Geometry: final body of the model. Coordinates: model frame, mm. Face numbers are marked on the shaded views. A direction names the side the tool comes from. Give positions to 0.01 mm unless a question says otherwise; leave off trailing zeros. Order: outer loops, then holes, each group sorted by start corner. A loop starts at its lowest first (then second) coordinate and runs counter-clockwise, first axis right, second up. Notation, with made-up numbers: (74.25, 76) - (111.25, 76) arc R27 cw to (111.25, 101) - close; hole circle Ø5 at (12.25, 17). An arc over 180 degrees is marked (long way). Use one line per item in the form item = value.
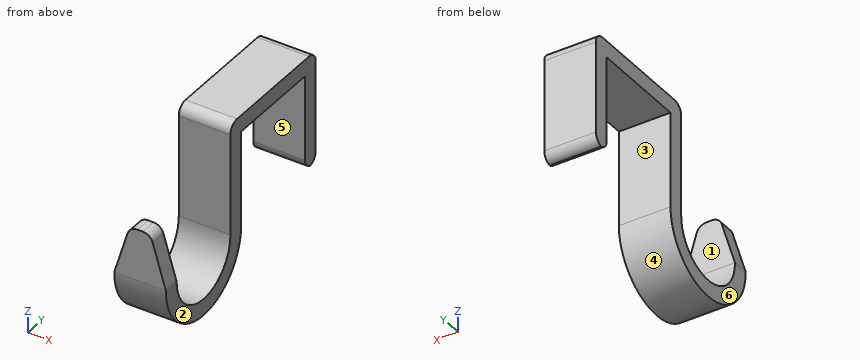
from build123d import *

# Parameters (mm, degrees)
F0_W        = 3.2
F0_H        = 10
F1_DEPTH    = 10
F2_SIZE2    = 10
F2_SIZE     = 3
F3_T1_DEPTH = 10.6403065089
F3_T3_DEPTH = 4.667688363
F3_T5_DEPTH = 20


# Not quite as in the source:
# - a fillet or chamfer that OpenCascade refuses, or shapes differently, is made with other operations: its cross-section is extruded or revolved along the edge and cut away or added


with BuildPart() as f1:
    # F0 (on Right) → F1 (new body)
    with BuildSketch(Plane.YZ):
        with Locations((-30.3, 5)):
            Rectangle(F0_W, F0_H)
        with BuildLine():
            Line((-9.5, 0), (-12.7, 0))
            ThreePointArc((-12.7, 0), (-20.7, -8), (-28.7, 0))
            Line((-28.7, 0), (-31.9, 0))
            ThreePointArc((-31.9, 0), (-20.7, -11.2), (-9.5, 0))
        make_face()
        Polygon((-12.7, 21.7), (-12.7, 0), (-9.5, 0), (-9.5, 18.5), (9.5, 18.5), (9.5, 0), (12.7, 0), (12.7, 21.7), align=None)
    extrude(amount=F1_DEPTH)

    # F2
    f2_edges = [f1.edges().sort_by_distance(p)[0] for p in [
        (10, -30.3, 10),
        (0, -30.3, 10),
    ]]
    f2_side = f1.faces().sort_by_distance((5, -30.3, 10))[0]
    chamfer(f2_edges, length=F2_SIZE, length2=F2_SIZE2, reference=f2_side)

    # F3: fillet of radius 2 on 8 edges, made by hand

    # F3_s2 → F3_t1 (cut)
    with BuildSketch(Plane.XZ.offset(24.9798467455)):
        with BuildLine():
            ThreePointArc((5.5119386982, 10), (6.7057997575, 9.6045858566), (7.4275912687, 8.5746957711))
            Line((7.4275912687, 8.5746957711), (7, 10))
            Line((7, 10), (5.5119386982, 10))
        make_face()
        with BuildLine():
            ThreePointArc((4.4880613018, 10), (3.2942002425, 9.6045858566), (2.5724087313, 8.5746957711))
            Line((2.5724087313, 8.5746957711), (3, 10))
            Line((3, 10), (4.4880613018, 10))
        make_face()
    extrude(amount=F3_T1_DEPTH, mode=Mode.SUBTRACT)

    # F3_s4 → F3_t3 (cut)
    with BuildSketch(Plane.XZ.offset(27.9661558185)):
        with BuildLine():
            ThreePointArc((9.9156525704, 0.2811580985), (9.978800791, -0.0031113832), (10, -0.2935376726))
            Line((10, -0.2935376726), (10, 0))
            Line((10, 0), (9.9156525704, 0.2811580985))
        make_face()
        with BuildLine():
            ThreePointArc((0.0843474296, 0.2811580985), (0.021199209, -0.0031113832), (0, -0.2935376726))
            Line((0, -0.2935376726), (0, 0))
            Line((0, 0), (0.0843474296, 0.2811580985))
        make_face()
    extrude(amount=F3_T3_DEPTH, mode=Mode.SUBTRACT)

    # F3_s6 → F3_t5 (cut)
    with BuildSketch(Plane.YZ.offset(-5)):
        with BuildLine():
            ThreePointArc((-12.7, 19.7), (-12.1142135624, 21.1142135624), (-10.7, 21.7))
            Line((-10.7, 21.7), (-12.7, 21.7))
            Line((-12.7, 21.7), (-12.7, 19.7))
        make_face()
        with BuildLine():
            ThreePointArc((10.7, 21.7), (12.1142135624, 21.1142135624), (12.7, 19.7))
            Line((12.7, 19.7), (12.7, 21.7))
            Line((12.7, 21.7), (10.7, 21.7))
        make_face()
        with BuildLine():
            ThreePointArc((9.5, 2), (10.0857864376, 0.5857864376), (11.5, 0))
            Line((11.5, 0), (9.5, 0))
            Line((9.5, 0), (9.5, 2))
        make_face()
        with BuildLine():
            ThreePointArc((12.7, 2), (12.1142135624, 0.5857864376), (10.7, 0))
            Line((10.7, 0), (12.7, 0))
            Line((12.7, 0), (12.7, 2))
        make_face()
    extrude(amount=F3_T5_DEPTH, mode=Mode.SUBTRACT)


solid = f1.part
(1) Cut plane C-C on z = -6.5. Output: boundary loops of the cut face in (x, y), plus the area to 3 significant figures.
Computed values:
outline = (0, -29.82) - (10, -29.82) - (10, -25.36) - (0, -25.36) - close; (0, -16.04) - (10, -16.04) - (10, -11.58) - (0, -11.58) - close
area = 89.1 mm²
(2) Pull-direction query (Y, two-part tool) for the marked faces 4, 5 and 6; classes: released by +Y, released by -Y, zero draft, split by the parting line, or undercut.
Computed values:
face_4 = split by the parting line
face_5 = undercut
face_6 = zero draft
(3) Cut plane D-D on z = 8. Output: boundary loops of the cut face in (x, y), plus the area to 3 significant figures.
Computed values:
outline = (0, -12.7) - (10, -12.7) - (10, -9.5) - (0, -9.5) - close; (0, 9.5) - (10, 9.5) - (10, 12.7) - (0, 12.7) - close; (2.4, -31.9) - (7.6, -31.9) - (7.6, -28.7) - (2.4, -28.7) - close
area = 80.6 mm²
(4) Ray query, line 1 along Y through (x, z) = (3, 15); line 2 along Z through (x, y) = (4.75, -1.5); line 3 along Y through (x, z) = (1, -2.5). Return the intervals inside material, ascending.
Computed values:
line_1 = -12.7 to -9.5, 9.5 to 12.7
line_2 = 18.5 to 21.7
line_3 = -31.62 to -28.3, -13.1 to -9.78
(5) Cut plane A-A on z = 4. Output: boundary loops of the cut face in (x, y).
Computed values:
outline = (0, -12.7) - (10, -12.7) - (10, -9.5) - (0, -9.5) - close; (0, 9.5) - (10, 9.5) - (10, 12.7) - (0, 12.7) - close; (1.2, -31.9) - (8.8, -31.9) - (8.8, -28.7) - (1.2, -28.7) - close
(6) Contact query for flat-ended pins moving along their axis: pin 1 Ø5 at (x, y) = (3.5, -1) entering from -Z; pin 2 Ø0.8 at (x, y) = (5, -30.5) entering from +Z; pin 3 Ø1 at (x, y) = (8.5, -12) entering from +Z. Output: stop coordinate, or through.
Computed values:
pin_1 = 18.5
pin_2 = 10
pin_3 = 21.53
(7) Cut plane B-B on x = 1.5. Output: boundary loops of the cut face in (y, z), plus the area to 3 significant figures.
Computed values:
outline = (-31.9, 0) arc R11.2 ccw to (-9.5, 0) - (-9.5, 18.5) - (9.5, 18.5) - (9.5, 2) arc R2 ccw to (11.1, 0.04) arc R2 ccw to (12.7, 2) - (12.7, 19.7) arc R2 ccw to (10.7, 21.7) - (-10.7, 21.7) arc R2 ccw to (-12.7, 19.7) - (-12.7, 0) arc R8 cw to (-28.7, 0) - (-28.7, 5) - (-31.9, 5) - close
area = 309 mm²
(8) Reachability of the marked faces 1, 2 and 3 from +Z, -Z, +X, -X, +Y, -Y: full face, straight path, thin tool, end or side. Return the list, or none.
Computed values:
face_1 = +Z, +X, -X
face_2 = +Z, -Z, +X, +Y, -Y
face_3 = -Z, +X, -X
